from build123d import *

# Parameters (mm, degrees)
IZIM1_W               = 120
IZIM1_H               = 12
IZIM2_W               = 120
IZIM2_H               = 8
KES_EKSTR_ZYON1_DEPTH = 18.3


with BuildPart() as part:
    # Çizim1 → Döndür1 (revolve)
    with BuildSketch(Plane.XY, mode=Mode.PRIVATE) as d_nd_r1_sk:
        with Locations((0, 21)):
            Rectangle(IZIM1_W, IZIM1_H)
    revolve(d_nd_r1_sk.sketch.rotate(Axis((-60, 0, 0), (1, 0, 0)), 180), axis=Axis((-60, 0, 0), (1, 0, 0)))

    # Çizim2 → Kes-Ekstrüzyon1 (cut)
    with BuildSketch(Plane(origin=(0, 0, 0), x_dir=(1, 0, 0), z_dir=(0, 1, 0))):
        Rectangle(IZIM2_W, IZIM2_H)
    extrude(amount=-KES_EKSTR_ZYON1_DEPTH, mode=Mode.SUBTRACT)

    # Çizim7 → M10 Dişli Delik4 (revolve, cut)
    with BuildSketch(Plane(origin=(-30.584904592, 0, -30), x_dir=(0, 1, 0), z_dir=(1, 0, 0))):
        Polygon((0, 0), (0, 37.113657631), (4.25, 34.56), (4.25, 0.775), (5.025, 0), align=None)
    m10_di_li_delik4 = revolve(axis=Axis((-30.584904592, 0, -36.35), (0, 0, 1)), mode=Mode.SUBTRACT)

    # Aynalama1: M10 Dişli Delik4 across plane
    add(m10_di_li_delik4.mirror(Plane.XY), mode=Mode.SUBTRACT)


solid = part.part
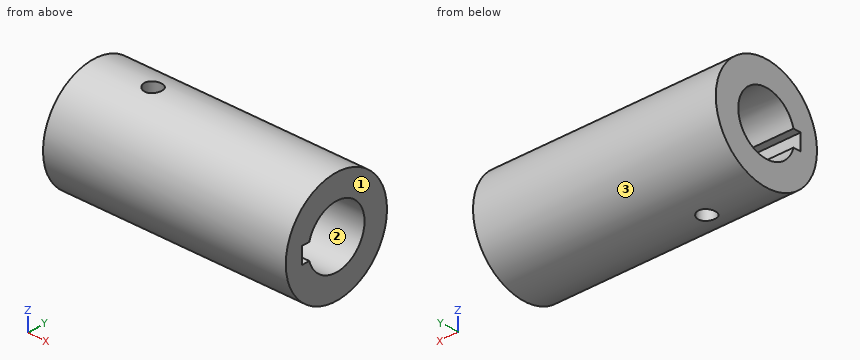
Could you check a few things on this model? Use its own coordinates, in mm. Face numbers are marked on the shaded views. Give positions to 0.01 mm unless a question says otherwise; leave off trailing zeros. Order: outer loops, then holes, each group sorted by start corner. A loop starts at its lowest first (then second) coordinate and runs counter-clockwise, first axis right, second up. Notation, with made-up numbers: (-21.75, -28) - (-5.75, -28) arc R10 ccw to (-5.75, -16) - close; hole circle Ø3 at (46, 47). An arc over 180 degrees is marked (long way). One line per question, with ' | ' between items. Start each with the question number.
Item 1: I'm going to push flat-ended pins straight in: pin 1 Ø10 at (x, y) = (-6.5, -6) entering from -Z; pin 2 Ø3 at (x, z) = (1, -13) entering from -Y; pin 3 Ø3 at (x, y) = (14.5, -16) entering from +Z; pin 4 Ø12 at (x, z) = (-20, 0.5) entering from -Y. Where does each tip first touch, or does it pass through?
Item 2: Thinking about a two-plate mould opening in Y: for the marked faces 1, 2 and 3, which applies, pulls with the +Y half, pulls with the -Y half, needs draft (parallel to the pull), parting line crosses it, or undercut?
Item 3: I need wall thicknesses on probe 1 along X at (y, z) = (0, -18); probe 2 along Z at (x, y) = (-42, 0); probe 3 along Y at (x, z) = (4, -2). Which ranges of each line are inside material? Lowest first, please. Write a range as [from, to].
Item 4: I want a section at D-D on y = 9. Write out the boundary of the cut face in (x, z), then the cut area to 3 significant figures.
Item 5: I want a section at B-B on x = -19. Write out the boundary of the cut face in (y, z).
Item 6: I want a section at A-A on y = 0. Write out the boundary of the cut face in (x, z), then the cut area to 3 significant figures.
Item 7: I want a section at C-C on z = 0. Write out the boundary of the cut face in (x, y), then the cut area to 3 significant figures.
Verdict:
1) pin 1: z = -26.98 | pin 2: y = -24.43 | pin 3: z = 22.78 | pin 4: y = -27
2) face 1: needs draft | face 2: undercut | face 3: parting line crosses it
3) probe 1: [-60, -34.83], [-26.33, 60] | probe 2: [-27, -15], [15, 27] | probe 3: [-26.93, -18.3], [14.87, 26.93]
4) outline: (-60, -25.46) - (60, -25.46) - (60, -12) - (-60, -12) - close; (-60, 12) - (60, 12) - (60, 25.46) - (-60, 25.46) - close | area: 3,230 mm^2
5) outline: circle Ø54 at (0, 0); hole (-18.3, -4) - (-14.46, -4) arc R15 ccw (long way) to (-14.46, 4) - (-18.3, 4) - close
6) outline: (-60, -27) - (-34.83, -27) - (-34.83, -15) - (-60, -15) - close; (-60, 15) - (-34.83, 15) - (-34.83, 27) - (-60, 27) - close; (-26.33, -27) - (60, -27) - (60, -15) - (-26.33, -15) - close; (-26.33, 15) - (60, 15) - (60, 27) - (-26.33, 27) - close | area: 2,680 mm^2
7) outline: (-60, -27) - (60, -27) - (60, -18.3) - (-60, -18.3) - close; (-60, 15) - (60, 15) - (60, 27) - (-60, 27) - close | area: 2,480 mm^2
